Part model, mm, in its own coordinate system. Round coordinates to 2 decimals unless told otherwise and drop trailing zeros.
1) Drill centre lines: L1, parallel to Y at x = 20, z = 4.75; L2, parallel to Y at x = 545, z = 6.25; L3, parallel to X at y = 105, z = 8.25. Where is each one in solid material? Low to high.
2) Flat gauge pin, fed straight in: pin 1 (3 mm diameter, centred on x = 545, y = 74, fed in from -Z). Where does the tip first touch, or does it go through?
3) Pull direction X, two halves, no side cores. Call faces 1 (the flat face through (296, 0, 6)), 2 (the flat face through (0, 59, 6)), 3 (the flat face through (600, 59, 6)): +X half, -X half, draft (parallel to the pull), parting line (faces both ways), or undercut.
```python
from build123d import *

# Parameters (mm, degrees)
SKETCH_1_W          = 600
SKETCH_1_H          = 120
EXTRUDE_1_DEPTH     = 12
SKETCH_4_R          = 3.5
CUT_EXTRUDE_1_DEPTH = 613
HOLE_WIZARD_M6_1_D  = 5


with BuildPart() as part:
    # 草图1 → 凸台-拉伸1 (new body)
    with BuildSketch(Plane.XY):
        with Locations((300, 60)):
            Rectangle(SKETCH_1_W, SKETCH_1_H)
    extrude(amount=EXTRUDE_1_DEPTH)

    # 草图4 → 切除-拉伸1 (cut, through all)
    with BuildSketch(Plane(origin=(0, 0, 0), x_dir=(-1, 0, 0), z_dir=(0, 0, -1))):
        with Locations((-20, 15)):
            Circle(SKETCH_4_R)
        with Locations(Location((-20, 105, 0), (0, 0, 180))):
            Circle(SKETCH_4_R)
    extrude(amount=-CUT_EXTRUDE_1_DEPTH, mode=Mode.SUBTRACT)

    # M6 螺纹孔1 (through all)
    with Locations(Plane(origin=(0, 0, 0), x_dir=(-1, 0, 0), z_dir=(0, 0, -1))):
        with Locations((-579, 74), (-545, 74)):
            Hole(HOLE_WIZARD_M6_1_D / 2)


solid = part.part
```
Completed:
1. L1: y = 0 to 11.5, 18.5 to 101.5, 108.5 to 120
1. L2: y = 0 to 71.5, 76.5 to 120
1. L3: x = 0 to 16.5, 23.5 to 600
2. pin 1: passes through
3. face 1: draft
3. face 2: -X half
3. face 3: +X half
